The listing builds one solid part. Answer for the finished solid, in the listing's coordinates (mm). Face numbers are marked on the shaded views. A direction names the side the tool comes from. Give positions to 0.01 mm unless a question says otherwise; leave off trailing zeros. Loops run counter-clockwise (first coordinate to the right, second up) from the corner with the lowest first, then second, coordinate; pieces in that order, holes last. Notation, with made-up numbers: M 32.5,-18 L 45.5,-18 A17 ccw 45.5,-14 Z; hole C 54.25,61 d9. An arc over 180 degrees is marked long. One line per item, written item: value. Start each with the question number.
Q1. A cutting plane is placed at A-A, the plane z = 3. Determine the outline of the cut face in (x, y).
Q2. A cutting plane is placed at D-D, the plane z = 6. Determine the outline of the cut face in (x, y), and give its area (3 significant figures).
Q3. A cutting plane is placed at C-C, the plane y = 17. Determine the outline of the cut face in (x, z), and give its area (3 significant figures).
Q4. Flat-ended cylindrical pins translate along their axes: pin 1 (1.5 mm diameter, centred on x = 12.5, z = 9, fed in from +Y); pin 2 (1.8 mm diameter, centred on y = 24.5, z = 5, fed in from +X); pin 3 (6 mm diameter, centred on y = 27.5, z = 7.5, fed in from -X). Find the tip coordinate at first contact, or state that the pin passes through.
Q5. Consider L1, parallel to Y at x = 7.5, z = 1.75; L2, parallel to X at y = 9.5, z = 11.25; L3, parallel to Y at x = 16, z = 9.75. Determine where each line is inside the solid, lowest interval first.
Q6. A cutting plane is placed at B-B, the plane x = 17. Determine the outline of the cut face in (y, z), and give its area (3 significant figures).
Q7. For the marked faces 1, 2 and 3, determine the directions among +Z, -Z, +X, -X, +Y, -Y from which every point of the face is accessible in a straight line to the end or side of a thin tool.
from build123d import *

# Parameters (mm, degrees)
SKETCH1_W           = 23
SKETCH1_H           = 29
BOSS_EXTRUDE1_DEPTH = 12
SKETCH3_W           = 34
SKETCH3_H           = 2
BOSS_EXTRUDE2_DEPTH = 12
SKETCH4_R           = 5
BOSS_EXTRUDE3_DEPTH = 2
SKETCH6_R           = 1.5
BOSS_EXTRUDE4_DEPTH = 3


with BuildPart() as part:
    # Sketch1 → Boss-Extrude1 (new body)
    with BuildSketch(Plane.XY):
        with Locations((11.5, 14.5)):
            Rectangle(SKETCH1_W, SKETCH1_H)
    extrude(amount=BOSS_EXTRUDE1_DEPTH)

    # Sketch3 → Boss-Extrude2 (add)
    with BuildSketch(Plane.XY.offset(12)):
        with Locations((11.5, 22)):
            Rectangle(SKETCH3_W, SKETCH3_H)
    extrude(amount=-BOSS_EXTRUDE2_DEPTH)

    # Sketch4 → Boss-Extrude3 (add)
    with BuildSketch(Plane(origin=(0, 29, 0), x_dir=(1, 0, 0), z_dir=(0, 1, 0))):
        with Locations(Location((17, -6, 0), (0, 0, 90))):
            Circle(SKETCH4_R)
    extrude(amount=BOSS_EXTRUDE3_DEPTH)

    # Sketch6 → Boss-Extrude4 (add)
    with BuildSketch(Plane(origin=(0, 31, 0), x_dir=(1, 0, 0), z_dir=(0, 1, 0))):
        with Locations(Location((17, -6, 0), (0, 0, 270))):
            Circle(SKETCH6_R)
    extrude(amount=BOSS_EXTRUDE4_DEPTH)


solid = part.part
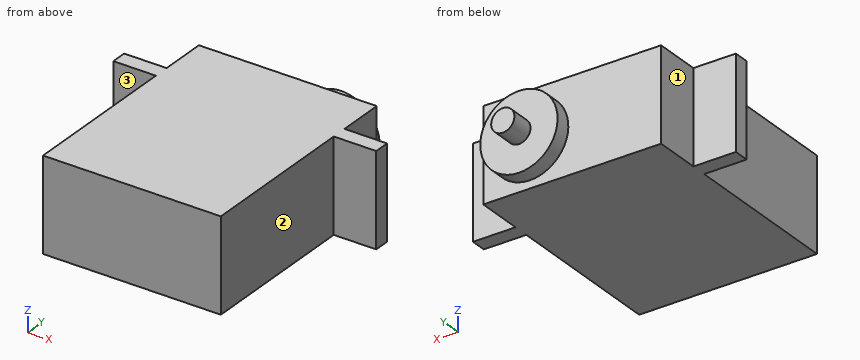
Answer block:
1. outline: M -5.5,21 L 0,21 L 0,0 L 23,0 L 23,21 L 28.5,21 L 28.5,23 L 23,23 L 23,29 L 21,29 L 21,31 L 13,31 L 13,29 L 0,29 L 0,23 L -5.5,23 Z
2. outline: M -5.5,21 L 0,21 L 0,0 L 23,0 L 23,21 L 28.5,21 L 28.5,23 L 23,23 L 23,29 L 22,29 L 22,31 L 18.5,31 L 18.5,34 L 15.5,34 L 15.5,31 L 12,31 L 12,29 L 0,29 L 0,23 L -5.5,23 Z
2. area: 718 mm^2
3. outline: M 0,0 L 23,0 L 23,12 L 0,12 Z
3. area: 276 mm^2
4. pin 1: y = 31
4. pin 2: x = 23
4. pin 3: x = 0
5. L1: 0 to 29
5. L2: 0 to 23
5. L3: 0 to 31
6. outline: M 0,0 L 29,0 L 29,1 L 31,1 L 31,4.5 L 34,4.5 L 34,7.5 L 31,7.5 L 31,11 L 29,11 L 29,12 L 0,12 Z
6. area: 377 mm^2
7. face 1: +Z, -Z, -X, +Y
7. face 2: +Z, -Z, +X, -Y
7. face 3: +Z, -Z, -X, -Y
